Work out the finished part from the listing and answer in its coordinate system (mm). Round coordinates to 2 decimals unless told otherwise and drop trailing zeros. Answer as a JSON object with one key per item and string values. Group by question number.
from build123d import *

# Parameters (mm, degrees)
SKETCH2_W                  = 25.4
SKETCH2_H                  = 2.41
BOSS_EXTRUDE1_DEPTH        = 8.51
SKETCH5_W                  = 1
SKETCH5_H                  = 1
CUT_EXTRUDE1_DEPTH         = 5
CHAMFER1_SIZE              = 0.5
LPATTERN3_COUNT            = 10
LPATTERN3_PITCH            = 2.54
CHAMFER1_OF_LPATTERN3_SIZE = 0.5
SKETCH11_W                 = 0.64
SKETCH11_H                 = 0.64
BOSS_EXTRUDE2_DEPTH        = 9.92
LPATTERN4_COUNT            = 10
LPATTERN4_PITCH            = 2.54


with BuildPart() as part:
    # Sketch2 → Boss-Extrude1 (new body)
    with BuildSketch(Plane(origin=(0, 0, 0), x_dir=(1, 0, 0), z_dir=(0, 1, 0))):
        with Locations((11.43, 0)):
            Rectangle(SKETCH2_W, SKETCH2_H)
    extrude(amount=BOSS_EXTRUDE1_DEPTH)

    # Sketch5 → Cut-Extrude1 (cut)
    with BuildSketch(Plane(origin=(0, 8.51, 0), x_dir=(1, 0, 0), z_dir=(0, 1, 0))):
        Rectangle(SKETCH5_W, SKETCH5_H)
    cut_extrude1 = extrude(amount=-CUT_EXTRUDE1_DEPTH, mode=Mode.SUBTRACT)

    # Chamfer1
    chamfer1_edges = [part.edges().sort_by_distance(p)[0] for p in [
        (0.5, 8.51, 0),
        (0, 8.51, -0.5),
        (-0.5, 8.51, 0),
        (0, 8.51, 0.5),
    ]]
    chamfer(chamfer1_edges, length=CHAMFER1_SIZE)

    # LPattern3: Cut-Extrude1 ×10
    with Locations(*[(i * LPATTERN3_PITCH, 0, 0) for i in range(1, LPATTERN3_COUNT)]):
        add(cut_extrude1, mode=Mode.SUBTRACT)

    # Chamfer1 of LPattern3
    chamfer1_of_lpattern3_edges = [part.edges().sort_by_distance(p)[0] for p in [
        (3.04, 8.51, 0),
        (2.54, 8.51, -0.5),
        (2.04, 8.51, 0),
        (2.54, 8.51, 0.5),
        (5.58, 8.51, 0),
        (5.08, 8.51, -0.5),
        (4.58, 8.51, 0),
        (5.08, 8.51, 0.5),
        (8.12, 8.51, 0),
        (7.62, 8.51, -0.5),
        (7.12, 8.51, 0),
        (7.62, 8.51, 0.5),
        (10.66, 8.51, 0),
        (10.16, 8.51, -0.5),
        (9.66, 8.51, 0),
        (10.16, 8.51, 0.5),
        (13.2, 8.51, 0),
        (12.7, 8.51, -0.5),
        (12.2, 8.51, 0),
        (12.7, 8.51, 0.5),
        (15.74, 8.51, 0),
        (15.24, 8.51, -0.5),
        (14.74, 8.51, 0),
        (15.24, 8.51, 0.5),
        (18.28, 8.51, 0),
        (17.78, 8.51, -0.5),
        (17.28, 8.51, 0),
        (17.78, 8.51, 0.5),
        (20.82, 8.51, 0),
        (20.32, 8.51, -0.5),
        (19.82, 8.51, 0),
        (20.32, 8.51, 0.5),
        (23.36, 8.51, 0),
        (22.86, 8.51, -0.5),
        (22.36, 8.51, 0),
        (22.86, 8.51, 0.5),
    ]]
    chamfer(chamfer1_of_lpattern3_edges, length=CHAMFER1_OF_LPATTERN3_SIZE)

    # Sketch11 → Boss-Extrude2 (add)
    with BuildSketch(Plane.XZ):
        Rectangle(SKETCH11_W, SKETCH11_H)
    boss_extrude2 = extrude(amount=BOSS_EXTRUDE2_DEPTH)

    # Sketch13 → Loft1 section 0
    with BuildSketch(Plane.XZ.offset(9.92)):
        with BuildLine():
            Line((0.32, -0.32), (0.32, 0.32))
            Line((0.32, 0.32), (-0.32, 0.32))
            Line((-0.32, 0.32), (-0.32, -0.32))
            Line((-0.32, -0.32), (0.32, -0.32))
        make_face()
    # Sketch14 → Loft1 section 1
    with BuildSketch(Plane(origin=(0, -10.49, 0), x_dir=(-1, 0, 0), z_dir=(0, -1, 0))):
        with BuildLine():
            Line((-0.22, 0.22), (0.22, 0.22))
            Line((0.22, 0.22), (0.22, -0.22))
            Line((0.22, -0.22), (-0.22, -0.22))
            Line((-0.22, -0.22), (-0.22, 0.22))
        make_face()
    loft1 = loft()

    # LPattern4: Boss-Extrude2, Loft1 ×10
    with Locations(*[(i * LPATTERN4_PITCH, 0, 0) for i in range(1, LPATTERN4_COUNT)]):
        add(boss_extrude2)
        add(loft1)


solid = part.part
1) Each of these flat-tipped pins is pushed along its axis until it touches: P1, Ø3, axis at x = 16.5, y = -7, coming from the +Z side; P2, Ø1.1, axis at x = 18, z = 0, coming from the +Y side; P3, Ø0.5, axis at x = 10.5, z = 0, coming from the +Y side. Where does it stop, or does it pass through?
2) For a pull along X with two mould halves and no side action, classify faces 1 (the face through (10.66, 6, 0)), 2 (the face through (15, 3.51, 0)) as released by +X, released by -X, zero draft, split by the parting line, or undercut.
3) A cutting plane is placed at A-A on y = -1.5. State how many separate pieces and enclosed holes the cut face has, plus the area to 3 significant figures.
4) Straight lines are drawn through the part: L1, parallel to Z at x = 18, y = 6.5 (3 decimals); L2, parallel to Y at x = 16.75, z = -0.55; L3, parallel to Y at x = 10.25, z = 0.9. For each, find the intervals that lie inside material, in ascending order.
Established:
{
 "1": {"P1": "stops at z = 0.32", "P2": "stops at y = 8.28", "P3": "stops at y = 8.1"},
 "2": {"face 1": "undercut", "face 2": "undercut"},
 "3": {"separate pieces": "10", "enclosed holes": "0", "area": "4.10 mm²"},
 "4": {"L1": "z = -1.205 to -0.5, 0.5 to 1.205", "L2": "y = 0 to 8.51", "L3": "y = 0 to 8.41"}
}
